```python
from build123d import *

# Parameters (mm, degrees)
SKETCH1_R           = 3.5
SKETCH1_R_2         = 7
BOSS_EXTRUDE1_DEPTH = 16
SKETCH3_R           = 23
CUT_EXTRUDE1_DEPTH  = 4
SKETCH4_R           = 45
SKETCH4_R_2         = 3.5
SKETCH4_R_3         = 40
SKETCH4_R_4         = 19
SKETCH4_R_5         = 14
SKETCH4_R_6         = 7
CUT_EXTRUDE2_DEPTH  = 6
FILLET1_R           = 4
FILLET2_R           = 2
CHAMFER1_SIZE       = 1
FILLET4_R           = 1


with BuildPart() as part:
    # Sketch1 → Boss-Extrude1 (new body)
    with BuildSketch(Plane.XY):
        Polygon((-53, -30.599564267), (0, -61.199128534), (53, -30.599564267), (53, 30.599564267), (0, 61.199128534), (-53, 30.599564267), align=None)
        with Locations((0, 51)):
            Circle(SKETCH1_R, mode=Mode.SUBTRACT)
        with Locations((44.167295593, 25.5)):
            Circle(SKETCH1_R, mode=Mode.SUBTRACT)
        with Locations((44.167295593, -25.5)):
            Circle(SKETCH1_R, mode=Mode.SUBTRACT)
        with Locations((0, -51)):
            Circle(SKETCH1_R, mode=Mode.SUBTRACT)
        with Locations((-44.167295593, -25.5)):
            Circle(SKETCH1_R, mode=Mode.SUBTRACT)
        with Locations((-44.167295593, 25.5)):
            Circle(SKETCH1_R, mode=Mode.SUBTRACT)
        Circle(SKETCH1_R_2, mode=Mode.SUBTRACT)
    extrude(amount=BOSS_EXTRUDE1_DEPTH)

    # Sketch3 → Cut-Extrude1 (cut)
    with BuildSketch(Plane.XY.offset(16)):
        Polygon((-53, 30.599564267), (-53, -30.599564267), (0, -61.199128534), (53, -30.599564267), (53, 30.599564267), (0, 61.199128534), align=None)
        Circle(SKETCH3_R, mode=Mode.SUBTRACT)
    extrude(amount=-CUT_EXTRUDE1_DEPTH, mode=Mode.SUBTRACT)

    # Sketch4 → Cut-Extrude2 (cut)
    # profile 1 of 3: a face of its own
    with BuildSketch(Plane(origin=(0, 0, 0), x_dir=(-1, 0, 0), z_dir=(0, 0, -1))):
        Polygon((0, -61.199128534), (53, -30.599564267), (53, 30.599564267), (0, 61.199128534), (-53, 30.599564267), (-53, -30.599564267), align=None)
        Circle(SKETCH4_R, mode=Mode.SUBTRACT)
        with Locations((0, 51)):
            Circle(SKETCH4_R_2, mode=Mode.SUBTRACT)
        with Locations((-44.167295593, 25.5)):
            Circle(SKETCH4_R_2, mode=Mode.SUBTRACT)
        with Locations((0, -51)):
            Circle(SKETCH4_R_2, mode=Mode.SUBTRACT)
        with Locations((44.167295593, 25.5)):
            Circle(SKETCH4_R_2, mode=Mode.SUBTRACT)
        with Locations((44.167295593, -25.5)):
            Circle(SKETCH4_R_2, mode=Mode.SUBTRACT)
        with Locations((-44.167295593, -25.5)):
            Circle(SKETCH4_R_2, mode=Mode.SUBTRACT)
    # profile 2 of 3: a face of its own
    with BuildSketch(Plane(origin=(0, 0, 0), x_dir=(-1, 0, 0), z_dir=(0, 0, -1))):
        Circle(SKETCH4_R_3)
        Circle(SKETCH4_R_4, mode=Mode.SUBTRACT)
    # profile 3 of 3: a face of its own
    with BuildSketch(Plane(origin=(0, 0, 0), x_dir=(-1, 0, 0), z_dir=(0, 0, -1))):
        Circle(SKETCH4_R_5)
        Circle(SKETCH4_R_6, mode=Mode.SUBTRACT)
    extrude(amount=-CUT_EXTRUDE2_DEPTH, mode=Mode.SUBTRACT)

    # Fillet1
    fillet1_edges = [part.edges().sort_by_distance(p)[0] for p in [
        (-23, 0, 12),
    ]]
    fillet(fillet1_edges, radius=FILLET1_R - 0.0001)  # a hair under: the kernel refuses the full size

    # Fillet2
    fillet2_edges = [part.edges().sort_by_distance(p)[0] for p in [
        (19, 0, 6),
        (-26.5, 45.899346401, 12),
        (26.5, 45.899346401, 12),
        (53, 0, 12),
        (26.5, -45.899346401, 12),
        (-26.5, -45.899346401, 12),
        (-53, 0, 12),
        (40, 0, 6),
    ]]
    fillet(fillet2_edges, radius=FILLET2_R)

    # Chamfer1
    chamfer1_edges = [part.edges().sort_by_distance(p)[0] for p in [
        (45, 0, 0),
    ]]
    chamfer(chamfer1_edges, length=CHAMFER1_SIZE)

    # Fillet4
    fillet4_edges = [part.edges().sort_by_distance(p)[0] for p in [
        (-26.5, 45.899346401, 6),
        (-53, 30.599564267, 8),
        (0, 61.199128534, 8),
        (-53, -30.599564267, 8),
        (0, -61.199128534, 8),
        (53, -30.599564267, 8),
        (53, 30.599564267, 8),
        (52.362858156, -30.231710252, 11.463768304),
        (0, -60.463420503, 11.463768304),
        (52.362858156, 30.231710252, 11.463768304),
        (-52.362858156, -30.231710252, 11.463768304),
        (0, 60.463420503, 11.463768304),
        (-52.362858156, 30.231710252, 11.463768304),
    ]]
    fillet(fillet4_edges, radius=FILLET4_R)


solid = part.part
```
Verification items for the finished model (mm, model axes). A direction names the side the tool comes from. Coordinates: 2 decimals unless noted, no trailing zeros. One line per question, with ' | ' between items. Start each with the question number.
1. Section check A-A (y = -25.5). Count the separate pieces of the cut face and the enclosed holes in it, plus the area to 3 significant figures.
2. Material ranges on line 1 along Y through (x, z) = (0, 1.15); line 2 along X through (y, z) = (-25.5, 7.85); line 3 along Y through (x, z) = (-17, 2.25), recorded low to high.
3. Draft check along X on faces 4 (the flat face through (-5.4, -4.8, 16)), 5 (the cylindrical face through (-25.835, -45.589, 11.43)), 6 (the cylindrical face through (8.67, -39.05, 1.97)). Enter one of: released by +X, released by -X, zero draft, split by the parting line, or undercut.
4. Access from +Z, -Z, +X, -X, +Y, -Y to the whole of each face (thin tool, end or side, straight path). Record for faces 1 (the cylindrical face through (-25.972, 45.857, 6.285)), 2 (the flat face through (6.4, 3.3, 6)), 3 (the flat face through (-12, -25, 12)).
5. Gauge pin test, flat ends, axial feed: P1, Ø4, axis at x = 44.17, y = -25.5, coming from the +Z side; P2, Ø1.5, axis at x = -24, z = 2.5, coming from the -Y side; P3, Ø11, axis at x = 0, y = -51, coming from the -Z side; P4, Ø11, axis at x = 44.17, y = 25.5, coming from the +Z side. Record the tip position at first contact, or that the pin passes through.
Computed values:
1) separate pieces: 3 | enclosed holes: 0 | area: 629 mm²
2) line 1: -45 to -40, -19 to -14, 14 to 19, 40 to 45 | line 2: -53 to -47.67, -40.67 to 40.67, 47.67 to 53 | line 3: -41.67 to -36.21, -8.49 to 8.49, 36.21 to 41.67
3) face 4: zero draft | face 5: released by -X | face 6: undercut
4) face 1: -Z, -X, +Y | face 2: -Z | face 3: +Z
5) P1: through | P2: y = -38.53 | P3: z = 6 | P4: z = 12
